from build123d import *

# Parameters (mm, degrees)
F1_DEPTH  = 6
F3_DEPTH  = 0.5
F5_DEPTH  = 0.5
F6_R      = 2.99999
F7_R      = 2.99999
F9_DEPTH  = 1.5
F11_DEPTH = 1.5


# Not quite as in the source:
# - a fillet or chamfer is up to 0.001 mm smaller than in the source, because OpenCascade refuses the exact size


with BuildPart() as f1:
    # F0 (on Top) → F1 (new body)
    with BuildSketch(Plane.XY):
        with BuildLine():
            ThreePointArc((-21.257927263, 3.0925971456), (-19.5135237331, 1.2849088277), (-19.5663380414, -1.2266427602))
            ThreePointArc((-19.5663380414, -1.2266427602), (-17.0596555887, 1.5276447909), (-13.757927263, 3.2504758611))
            Line((-13.757927263, 3.2504758611), (-13.757927263, 16.4425971456))
            Line((-13.757927263, 16.4425971456), (-21.257927263, 12.0925971456))
            Line((-21.257927263, 12.0925971456), (-21.257927263, 3.0925971456))
        make_face()
        with BuildLine():
            ThreePointArc((-19.937029438, -1.8621137259), (-13.1593751133, -17.2347921219), (0.092072737, -6.9074028544))
            ThreePointArc((0.092072737, -6.9074028544), (-0.2305379955, -4.3059550041), (-1.178825088, -1.8621137259))
            ThreePointArc((-1.178825088, -1.8621137259), (-1.3821012217, -1.5548376637), (-1.5495164847, -1.2266427602))
            ThreePointArc((-1.5495164847, -1.2266427602), (-4.0561989374, 1.5276447909), (-7.357927263, 3.2504758611))
            Line((-7.357927263, 3.2504758611), (-7.357927263, 1.1925971456))
            Line((-7.357927263, 1.1925971456), (-10.557927263, 1.1925971456))
            Line((-10.557927263, 1.1925971456), (-13.757927263, 1.1925971456))
            Line((-13.757927263, 1.1925971456), (-13.757927263, 3.2504758611))
            ThreePointArc((-13.757927263, 3.2504758611), (-17.0596555887, 1.5276447909), (-19.5663380414, -1.2266427602))
            ThreePointArc((-19.5663380414, -1.2266427602), (-19.7337533043, -1.5548376637), (-19.937029438, -1.8621137259))
        make_face()
        with BuildLine():
            ThreePointArc((-7.407927263, -6.9074028544), (-12.7853136237, -9.1347892152), (-10.557927263, -3.7574028544))
            ThreePointArc((-10.557927263, -3.7574028544), (-8.3305409023, -4.6800164937), (-7.407927263, -6.9074028544))
        make_face(mode=Mode.SUBTRACT)
        with BuildLine():
            ThreePointArc((-7.357927263, 3.2504758611), (-4.0561989374, 1.5276447909), (-1.5495164847, -1.2266427602))
            ThreePointArc((-1.5495164847, -1.2266427602), (-1.6023307929, 1.2849088277), (0.142072737, 3.0925971456))
            Line((0.142072737, 3.0925971456), (0.142072737, 12.0925971456))
            Line((0.142072737, 12.0925971456), (-7.357927263, 16.4425971456))
            Line((-7.357927263, 16.4425971456), (-7.357927263, 3.2504758611))
        make_face()
    extrude(amount=F1_DEPTH)

    # F2 (on face) → F3 (join)
    with BuildSketch(Plane.YZ.offset(-13.757927263)):
        with BuildLine():
            ThreePointArc((11.9425971456, 0), (14.0639174891, 0.8786796564), (14.9425971456, 3))
            ThreePointArc((14.9425971456, 3), (14.0639174891, 5.1213203436), (11.9425971456, 6))
            ThreePointArc((11.9425971456, 6), (8.9425971456, 3), (11.9425971456, 0))
        make_face()
    extrude(amount=F3_DEPTH)

    # F4 (on face) → F5 (join)
    with BuildSketch(Plane(origin=(-7.357927263, 0, 0), x_dir=(0, -1, 0), z_dir=(-1, 0, 0))):
        with BuildLine():
            ThreePointArc((-11.9425971456, 0), (-9.821276802, 0.8786796564), (-8.9425971456, 3))
            ThreePointArc((-8.9425971456, 3), (-9.821276802, 5.1213203436), (-11.9425971456, 6))
            ThreePointArc((-11.9425971456, 6), (-14.9425971456, 3), (-11.9425971456, 0))
        make_face()
    extrude(amount=F5_DEPTH)

    # F6 (radius 3 in the source; OpenCascade refuses exactly that, so slightly less here)
    f6_edges = [f1.edges().sort_by_distance(p)[0] for p in [
        (-10.557927, 1.192597, 0),
        (-10.557927, 1.192597, 6),
    ]]
    fillet(f6_edges, radius=F6_R)

    # F7 (radius 3 in the source; OpenCascade refuses exactly that, so slightly less here)
    f7_edges = [f1.edges().sort_by_distance(p)[0] for p in [
        (-3.607927, 14.267597, 6),
        (-3.607927, 14.267597, 0),
        (-17.507927, 14.267597, 6),
        (-17.507927, 14.267597, 0),
    ]]
    fillet(f7_edges, radius=F7_R)

    # F8 (on face) → F9 (cut)
    with BuildSketch(Plane.XY.offset(6)):
        with BuildLine():
            ThreePointArc((-10.3315528874, -12.4037176265), (-8.5586184667, -13.6203290978), (-9.5390766145, -15.534001419))
            ThreePointArc((-9.5390766145, -15.534001419), (-12.5657731947, -13.9373786235), (-10.6819972396, -11.0805473911))
            ThreePointArc((-10.6819972396, -11.0805473911), (-9.6634977684, -11.1643464321), (-8.7690087855, -11.6585659294))
            Line((-8.7690087855, -11.6585659294), (-6.4111007419, -9.9150485592))
            Line((-6.4111007419, -9.9150485592), (-6.7083751907, -9.5130188313))
            Line((-6.7083751907, -9.5130188313), (-8.7669816313, -11.0352224208))
            ThreePointArc((-8.7669816313, -11.0352224208), (-9.7165335049, -10.6334325304), (-10.7464416358, -10.5847178642))
            ThreePointArc((-10.7464416358, -10.5847178642), (-10.7524542145, -10.5858192208), (-10.7585352096, -10.5864401769))
            ThreePointArc((-10.7585352096, -10.5864401769), (-12.1066928754, -11.1876295757), (-12.9640803834, -12.3892303605))
            Line((-12.9640803834, -12.3892303605), (-14.113424494, -15.4995148073))
            Line((-14.113424494, -15.4995148073), (-14.3623176984, -16.1730543119))
            Line((-14.3623176984, -16.1730543119), (-13.6445064842, -16.1730543119))
            Line((-13.6445064842, -16.1730543119), (-10.3284124834, -16.1730543119))
            ThreePointArc((-10.3284124834, -16.1730543119), (-9.8409208438, -16.1304430443), (-9.3682147094, -16.0039016311))
            ThreePointArc((-9.3682147094, -16.0039016311), (-9.361792524, -16.0016997739), (-9.355524465, -15.9990913118))
            ThreePointArc((-9.355524465, -15.9990913118), (-8.073910256, -13.497618257), (-10.3914165669, -11.9073142221))
            ThreePointArc((-10.3914165669, -11.9073142221), (-10.4058889802, -11.9084903608), (-10.4200689017, -11.9116150811))
            ThreePointArc((-10.4200689017, -11.9116150811), (-11.528535351, -14.0033516217), (-9.233119707, -14.5822528616))
            ThreePointArc((-9.233119707, -14.5822528616), (-9.1701495178, -14.5297943991), (-9.1224097378, -14.46317572))
            ThreePointArc((-9.1224097378, -14.46317572), (-9.1661029488, -13.263231915), (-10.3166224177, -12.9196053972))
            Line((-10.3166224177, -12.9196053972), (-10.1537286636, -13.392326906))
            ThreePointArc((-10.1537286636, -13.392326906), (-9.561565173, -13.5691888225), (-9.5390766145, -14.1867906375))
            ThreePointArc((-9.5390766145, -14.1867906375), (-11.0716295176, -13.8002825215), (-10.3315528874, -12.4037176265))
        make_face()
        with BuildLine():
            ThreePointArc((-13.0496571933, -14.0633096924), (-12.6340614687, -14.9692167321), (-11.9283702953, -15.6730543119))
            Line((-11.9283702953, -15.6730543119), (-13.6445064842, -15.6730543119))
            Line((-13.6445064842, -15.6730543119), (-13.0496571933, -14.0633096924))
        make_face(mode=Mode.SUBTRACT)
    extrude(amount=-F9_DEPTH, mode=Mode.SUBTRACT)

    # F10 (on face) → F11 (cut)
    with BuildSketch(Plane(origin=(0, 0, 0), x_dir=(1, 0, 0), z_dir=(0, 0, -1))):
        with BuildLine():
            Line((-6.4111007419, 9.9150485592), (-8.7690087855, 11.6585659294))
            ThreePointArc((-8.7690087855, 11.6585659294), (-9.6634977684, 11.1643464321), (-10.6819972396, 11.0805473911))
            ThreePointArc((-10.6819972396, 11.0805473911), (-12.5657731947, 13.9373786235), (-9.5390766145, 15.534001419))
            ThreePointArc((-9.5390766145, 15.534001419), (-8.5586184667, 13.6203290978), (-10.3315528874, 12.4037176265))
            ThreePointArc((-10.3315528874, 12.4037176265), (-11.0716295176, 13.8002825215), (-9.5390766145, 14.1867906375))
            ThreePointArc((-9.5390766145, 14.1867906375), (-9.561565173, 13.5691888225), (-10.1537286636, 13.392326906))
            Line((-10.1537286636, 13.392326906), (-10.3166224177, 12.9196053972))
            ThreePointArc((-10.3166224177, 12.9196053972), (-9.1661029488, 13.263231915), (-9.1224097378, 14.46317572))
            ThreePointArc((-9.1224097378, 14.46317572), (-9.1701495178, 14.5297943991), (-9.233119707, 14.5822528616))
            ThreePointArc((-9.233119707, 14.5822528616), (-11.528535351, 14.0033516217), (-10.4200689017, 11.9116150811))
            ThreePointArc((-10.4200689017, 11.9116150811), (-10.4058889802, 11.9084903608), (-10.3914165669, 11.9073142221))
            ThreePointArc((-10.3914165669, 11.9073142221), (-8.073910256, 13.497618257), (-9.355524465, 15.9990913118))
            ThreePointArc((-9.355524465, 15.9990913118), (-9.361792524, 16.0016997739), (-9.3682147094, 16.0039016311))
            ThreePointArc((-9.3682147094, 16.0039016311), (-9.8409208438, 16.1304430443), (-10.3284124834, 16.1730543119))
            Line((-10.3284124834, 16.1730543119), (-14.3623176984, 16.1730543119))
            Line((-14.3623176984, 16.1730543119), (-12.9640803834, 12.3892303605))
            ThreePointArc((-12.9640803834, 12.3892303605), (-12.1066928754, 11.1876295757), (-10.7585352096, 10.5864401769))
            ThreePointArc((-10.7585352096, 10.5864401769), (-10.7524542145, 10.5858192208), (-10.7464416358, 10.5847178642))
            ThreePointArc((-10.7464416358, 10.5847178642), (-9.7165335049, 10.6334325304), (-8.7669816313, 11.0352224208))
            Line((-8.7669816313, 11.0352224208), (-6.7083751907, 9.5130188313))
            Line((-6.7083751907, 9.5130188313), (-6.4111007419, 9.9150485592))
        make_face()
        with BuildLine():
            ThreePointArc((-11.9283702953, 15.6730543119), (-12.6340614687, 14.9692167321), (-13.0496571933, 14.0633096924))
            Line((-13.0496571933, 14.0633096924), (-13.6445064842, 15.6730543119))
            Line((-13.6445064842, 15.6730543119), (-11.9283702953, 15.6730543119))
        make_face(mode=Mode.SUBTRACT)
    extrude(amount=-F11_DEPTH, mode=Mode.SUBTRACT)


solid = f1.part
Part model, mm, in its own coordinate system. A direction names the side the tool comes from. Coordinates: 2 decimals unless noted, no trailing zeros. Loops run counter-clockwise (first coordinate to the right, second up) from the corner with the lowest first, then second, coordinate; pieces in that order, holes last. Notation, with made-up numbers: (68, 4) -> (83, 4) arc R21 cw to (83, 19) -> close; hole circle Ø6 at (89.5, -3). An arc over 180 degrees is marked (long way). Use a Markdown table: item, result. Add a question column.
Item 1: Flat gauge pins, fed straight in: P1, Ø1.6, axis at x = -12.5, z = 5, coming from the -Y side; P2, Ø3, axis at y = 12, z = 4, coming from the +X side; P3, Ø2, axis at x = -12, y = 13, coming from the +Z side (3 decimals); P4, Ø1.3, axis at y = 14.5, z = 4.5, coming from the +X side. Where does each tip first touch, or does it go through?
Item 2: Probe probe 1 along X at (y, z) = (10.5, 2.75); probe 2 along X at (y, z) = (4, 5.75); probe 3 along X at (y, z) = (0, 2.75). List the from-to ranges inside material, lowest first.
Item 3: Pull direction Y, two halves, no side cores. Call faces 1 (the cylindrical face through (-17.871, 13.014, 0.855)), 2 (the flat face through (-11.3, -14.1, 4.5)), 3 (the flat face through (-11, -2, 0)): +Y half, -Y half, draft (parallel to the pull), parting line (faces both ways), or undercut.
Item 4: Band-saw the part on A-A on y = 4. Write the cut outline in (x, z).
Item 5: Which spindle directions (+Z, -Z, +X, -X, +Y, -Y) get a long thin tool onto all of the face, cutting with end or side? Do faces 4 (the flat face through (-13.35, -14.88, 5.26)), 5 (the cylindrical face through (-3.37, 13.09, 5.14)), 6 (the cylindrical face through (-11.51, -14.04, 0.74)). Say none if no direction does.
Item 6: Band-saw the part on B-B on z = 2.25. Write the cut outline in (x, y).
Geometry says:
| question | item | result |
|---|---|---|
| 1 | P1 | y = -17.5 |
| 1 | P2 | x = 0.14 |
| 1 | P3 | through |
| 1 | P4 | x = -3.51 |
| 2 | probe 1 | -21.26 to -13.26, -7.86 to 0.14 |
| 2 | probe 2 | -21.26 to -13.76, -7.36 to 0.14 |
| 2 | probe 3 | -19.29 to -1.83 |
| 3 | face 1 | +Y half |
| 3 | face 2 | undercut |
| 3 | face 3 | draft |
| 4 | outline | (-21.26, 0) -> (-13.76, 0) -> (-13.76, 6) -> (-21.26, 6) -> close; (-7.36, 0) -> (0.14, 0) -> (0.14, 6) -> (-7.36, 6) -> close |
| 5 | face 4 | +Z |
| 5 | face 5 | +Z, +X, +Y |
| 5 | face 6 | -Z |
| 6 | outline | (-21.26, 3.09) arc R3.27 cw to (-19.94, -1.86) arc R10.65 ccw (long way) to (-1.18, -1.86) arc R3.27 cw to (0.14, 3.09) -> (0.14, 11.98) -> (-7.36, 16.33) -> (-7.36, 14.85) -> (-7.86, 14.85) -> (-7.86, 9.04) -> (-7.36, 9.04) -> (-7.36, 1.1) -> (-13.76, 1.1) -> (-13.76, 9.04) -> (-13.26, 9.04) -> (-13.26, 14.85) -> (-13.76, 14.85) -> (-13.76, 16.33) -> (-21.26, 11.98) -> close; hole circle Ø6.3 at (-10.56, -6.91) |
